Read the model definition and answer for the solid it produces. Units are mm, in the model's axes. Face numbers are marked on the shaded views. Coordinates: 2 decimals unless noted, no trailing zeros. Order: outer loops, then holes, each group sorted by start corner. A loop starts at its lowest first (then second) coordinate and runs counter-clockwise, first axis right, second up. Notation, with made-up numbers: (-26, 44.5) -> (31, 44.5) arc R27 ccw to (31, 63.5) -> close; hole circle Ø9 at (87, 77). An arc over 180 degrees is marked (long way). Use CSV: the item, a comma, the result in double quotes.
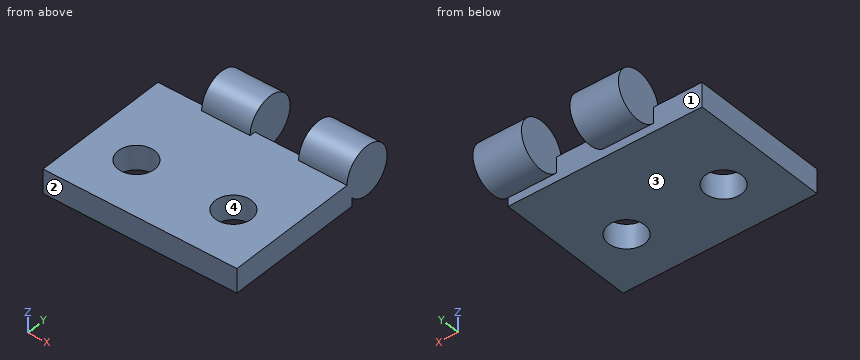
```python
from build123d import *

# Parameters (mm, degrees)
SKETCH1_W             = 16
SKETCH1_H             = 11.5
BOSS_EXTRUDE1_DEPTH   = 2
SKETCH2_R             = 2
BOSS_EXTRUDE2_DEPTH   = 4
LPATTERN1_COUNT       = 2
LPATTERN1_PITCH       = 8
F_3_0MM_DOWEL_HOLE1_D = 3


with BuildPart() as part:
    # Sketch1 → Boss-Extrude1 (new body)
    with BuildSketch(Plane.XY):
        with Locations((8, 5.75)):
            Rectangle(SKETCH1_W, SKETCH1_H)
    extrude(amount=BOSS_EXTRUDE1_DEPTH)

    # Sketch2 → Boss-Extrude2 (add)
    with BuildSketch(Plane(origin=(16, 0, 0), x_dir=(0, 0, -1), z_dir=(1, 0, 0))):
        with Locations((-2, 13.01793751)):
            Circle(SKETCH2_R)
    boss_extrude2 = extrude(amount=-BOSS_EXTRUDE2_DEPTH)

    # LPattern1: Boss-Extrude2 ×2
    with Locations(*[(-i * LPATTERN1_PITCH, 0, 0) for i in range(1, LPATTERN1_COUNT)]):
        add(boss_extrude2)

    # Ø3.0mm Dowel Hole1 (through all)
    with Locations(Plane.XY.offset(2)):
        with Locations((4, 4.5), (12, 4.5)):
            Hole(F_3_0MM_DOWEL_HOLE1_D / 2)


solid = part.part
```
Item 1: Straight lines are drawn through the part: line 1 along X through (y, z) = (13.25, 0.6); line 2 along Y through (x, z) = (9.5, 1); line 3 along Z through (x, y) = (10, 3). For each, find the intervals that lie inside material, in ascending order.
Return value:
line 1,"x = 4 to 8, 12 to 16"
line 2,"y = 0 to 11.5"
line 3,"z = 0 to 2"
Item 2: Find section C-C, the plane z = 1.15. Give the vertices of the cut face in (x, y), then the cut area to 3 significant figures.
Return value:
outline,"(0, 0) -> (16, 0) -> (16, 14.83) -> (12, 14.83) -> (12, 11.5) -> (8, 11.5) -> (8, 14.83) -> (4, 14.83) -> (4, 11.5) -> (0, 11.5) -> close; hole circle Ø3 at (4, 4.5); hole circle Ø3 at (12, 4.5)"
area,"196 mm^2"
Item 3: Find section D-D, the plane y = 11.25. Give the vertices of the cut face in (x, z).
Return value:
outline,"(0, 0) -> (16, 0) -> (16, 2.94) -> (12, 2.94) -> (12, 2) -> (8, 2) -> (8, 2.94) -> (4, 2.94) -> (4, 2) -> (0, 2) -> close"
Item 4: Each of these flat-tipped pins is pushed along its axis until it touches: P1, Ø3, axis at x = 3, y = 3.5, coming from the +Z side; P2, Ø1.2, axis at y = 13, z = 1, coming from the -X side; P3, Ø1.5, axis at x = 4.5, z = 1, coming from the +Y side. Where does it stop, or does it pass through?
Return value:
P1,"stops at z = 2"
P2,"stops at x = 4"
P3,"stops at y = 15"
Item 5: The mould has two halves that part along Y. Classify the marked faces 1, 2, 3 and 4: +Y half, -Y half, draft (parallel to the pull), parting line (faces both ways), or undercut.
Return value:
face 1,"undercut"
face 2,"-Y half"
face 3,"draft"
face 4,"undercut"
Item 6: Find section B-B, the plane z = 2.25. Give the vertices of the cut face in (x, y).
Return value:
outline,"(4, 11.03) -> (8, 11.03) -> (8, 15) -> (4, 15) -> close; (12, 11.03) -> (16, 11.03) -> (16, 15) -> (12, 15) -> close"
Item 7: Find section A-A, the plane y = 4.5. Give the vertices of the cut face in (x, z).
Return value:
outline,"(0, 0) -> (2.5, 0) -> (2.5, 2) -> (0, 2) -> close; (5.5, 0) -> (10.5, 0) -> (10.5, 2) -> (5.5, 2) -> close; (13.5, 0) -> (16, 0) -> (16, 2) -> (13.5, 2) -> close"
